The listing builds one solid part. Answer for the finished solid, in the listing's coordinates (mm). A direction names the side the tool comes from. Give positions to 0.01 mm unless a question says otherwise; leave off trailing zeros. Write each loop counter-clockwise with the first axis right and the second up, starting at its lowest first coordinate (ties: lowest second). Pieces come first, ordered by that corner, then holes.
```python
from build123d import *

# Parameters (mm, degrees)
SKETCH_W          = 292.1
SKETCH_H          = 609.6
PAD_DEPTH         = 19.05
BOX_W             = 3.175
BOX_H             = 609.6
BOX_DEPTH         = 6.35
BOX001_W          = 3.175
BOX001_H          = 609.6
BOX001_DEPTH      = 6.35
CYLINDER_R        = 6.35
CYLINDER_DEPTH    = 6.35
CYLINDER001_R     = 6.35
CYLINDER001_DEPTH = 6.35
CYLINDER002_R     = 6.35
CYLINDER002_DEPTH = 6.35
CYLINDER003_R     = 6.35
CYLINDER003_DEPTH = 6.35


with BuildPart() as part:
    # Sketch → Pad (new body)
    with BuildSketch(Plane.YZ):
        with Locations((0, 304.8)):
            Rectangle(SKETCH_W, SKETCH_H)
    extrude(amount=PAD_DEPTH)

    # Box → Box (cut)
    with BuildSketch(Plane(origin=(12.7, -136.525, 0), x_dir=(0, 1, 0), z_dir=(1, 0, 0))):
        with Locations((1.5875, 304.8)):
            Rectangle(BOX_W, BOX_H)
    extrude(amount=BOX_DEPTH, mode=Mode.SUBTRACT)

    # Box001 → Box001 (cut)
    with BuildSketch(Plane(origin=(12.7, 133.35, 0), x_dir=(0, 1, 0), z_dir=(1, 0, 0))):
        with Locations((1.5875, 304.8)):
            Rectangle(BOX001_W, BOX001_H)
    extrude(amount=BOX001_DEPTH, mode=Mode.SUBTRACT)

    # Cylinder → Cylinder (cut)
    with BuildSketch(Plane(origin=(12.7, -63.5, 444.5), x_dir=(0, 1, 0), z_dir=(1, 0, 0))):
        Circle(CYLINDER_R)
    extrude(amount=CYLINDER_DEPTH, mode=Mode.SUBTRACT)

    # Cylinder001 → Cylinder001 (cut)
    with BuildSketch(Plane(origin=(12.7, 38.1, 444.5), x_dir=(0, 1, 0), z_dir=(1, 0, 0))):
        Circle(CYLINDER001_R)
    extrude(amount=CYLINDER001_DEPTH, mode=Mode.SUBTRACT)

    # Cylinder002 → Cylinder002 (cut)
    with BuildSketch(Plane(origin=(12.7, 38.1, 190.5), x_dir=(0, 1, 0), z_dir=(1, 0, 0))):
        Circle(CYLINDER002_R)
    extrude(amount=CYLINDER002_DEPTH, mode=Mode.SUBTRACT)

    # Cylinder003 → Cylinder003 (cut)
    with BuildSketch(Plane(origin=(12.7, -63.5, 190.5), x_dir=(0, 1, 0), z_dir=(1, 0, 0))):
        Circle(CYLINDER003_R)
    extrude(amount=CYLINDER003_DEPTH, mode=Mode.SUBTRACT)


solid = part.part
```
Item 1: Consider probe 1 along Y at (x, z) = (14.75, 426.5) (3 decimals); probe 2 along Z at (x, y) = (14.5, 38.1); probe 3 along Z at (x, y) = (15.75, 36). Determine where each line is inside the solid, lowest interval first.
Conclusion:
probe 1: y = -146.05 to -136.525, -133.35 to 133.35, 136.525 to 146.05
probe 2: z = 0 to 184.15, 196.85 to 438.15, 450.85 to 609.6
probe 3: z = 0 to 184.51, 196.49 to 438.51, 450.49 to 609.6
Item 2: Which of the six approach directions +Z, -Z, +X, -X, +Y, -Y give full straight-line access (tool end or side, diameter ignored) to faces 4 (the face through (9, -2, 609.6)), 5 (the face through (12.7, 38, 445))?
Conclusion:
face 4: +Z, +X, -X, +Y, -Y
face 5: +X
Item 3: A cutting plane is placed at B-B, the plane z = 190.5. Give the vertices of the cut face in (x, y) (3 decimals).
Conclusion:
outline: (0, -146.05) - (19.05, -146.05) - (19.05, -136.525) - (12.7, -136.525) - (12.7, -133.35) - (19.05, -133.35) - (19.05, -69.85) - (12.7, -69.85) - (12.7, -57.15) - (19.05, -57.15) - (19.05, 31.75) - (12.7, 31.75) - (12.7, 44.45) - (19.05, 44.45) - (19.05, 133.35) - (12.7, 133.35) - (12.7, 136.525) - (19.05, 136.525) - (19.05, 146.05) - (0, 146.05) - close
Item 4: Determine the mould class of faces 1 (the face through (12.7, -64, 445)), 2 (the face through (9, -2, 0)), 3 (the face through (9, 146.05, 301)) for opening direction Y: pulls with the +Y half, pulls with the -Y half, needs draft (parallel to the pull), parting line crosses it, or undercut.
Conclusion:
face 1: undercut
face 2: needs draft
face 3: pulls with the +Y half
Item 5: This flat-tipped pin is pushed along its axis until it touches: P1, Ø4, axis at y = 38, z = 442.5, coming from the +X side. Where does it stop, or does it pass through?
Conclusion:
P1: stops at x = 12.7
Item 6: A cutting plane is placed at A-A, the plane x = 16. Give the vertices of the cut face in (y, z) (3 decimals), plus the area to 3 significant figures.
Conclusion:
outline: (-146.05, 0) - (-136.525, 0) - (-136.525, 609.6) - (-146.05, 609.6) - close; (-133.35, 0) - (133.35, 0) - (133.35, 609.6) - (-133.35, 609.6) - close; (136.525, 0) - (146.05, 0) - (146.05, 609.6) - (136.525, 609.6) - close; hole circle Ø12.7 at (-63.5, 190.5); hole circle Ø12.7 at (-63.5, 444.5); hole circle Ø12.7 at (38.1, 190.5); hole circle Ø12.7 at (38.1, 444.5)
area: 174,000 mm2
